Could you check a few things on this drawing? It's one solid part, dimensions in mm from its lowest x, y, z. A direction names the side the tool comes from. Round coordinates to 2 decimals unless told otherwise and drop trailing zeros. Loops run counter-clockwise (first coordinate to the right, second up) from the corner with the lowest first, then second, coordinate; pieces in that order, holes last. Notation, with made-up numbers: (49, 66) -> (75, 66) arc R24 ccw to (75, 81) -> close; hole circle Ø7 at (2.5, -30.75). An arc over 180 degrees is marked (long way). Write each question's results on one line, items separated by ' | '.
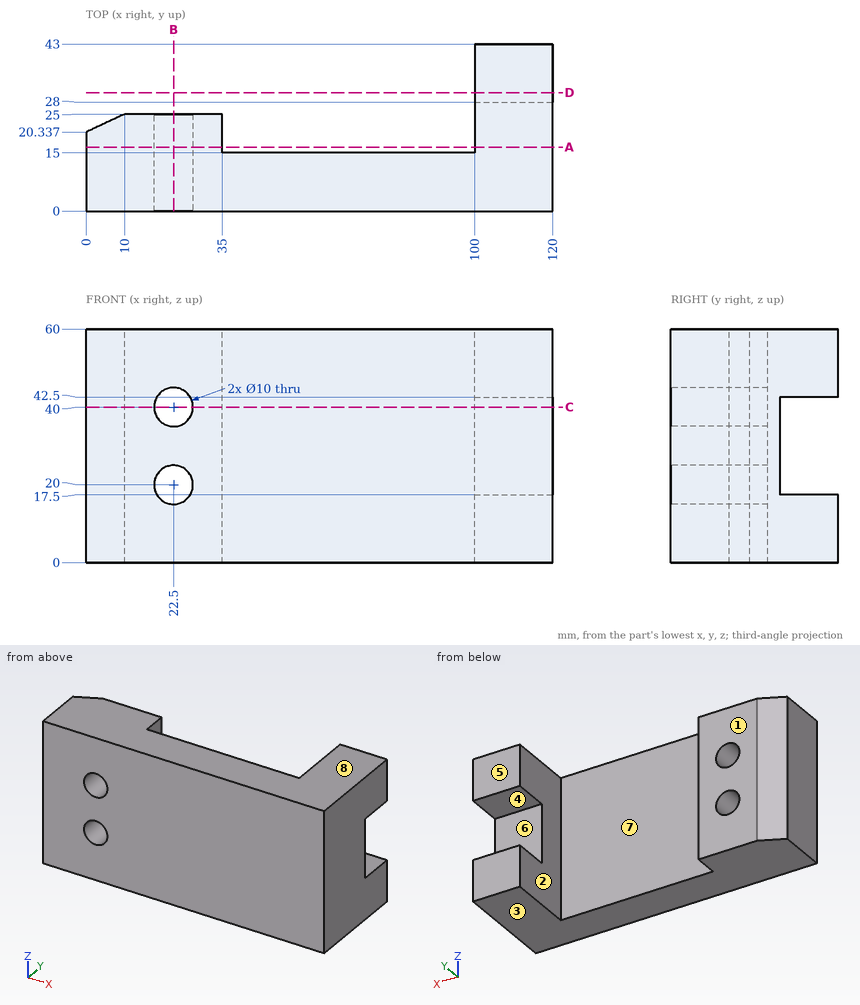
1) I want a section at C-C, the plane z = 40. Write out the boundary of the cut face in (x, y), plus the area to 3 significant figures.
Model answer:
outline: (0, 0) -> (17.5, 0) -> (17.5, 25) -> (10, 25) -> (0, 20.34) -> close; (27.5, 0) -> (120, 0) -> (120, 28) -> (100, 28) -> (100, 15) -> (35, 15) -> (35, 25) -> (27.5, 25) -> close | area: 2,140 mm2
2) I'm going to push flat-ended pins straight in: pin 1 (1.5 mm diameter, centred on x = 91.5, z = 8, fed in from +Y); pin 2 (5 mm diameter, centred on y = 6, z = 11.5, fed in from -X); pin 3 (14 mm diameter, centred on y = 27.5, z = 40, fed in from -X); pin 4 (10 mm diameter, centred on x = 111, z = 32.5, fed in from +Y). Where does each tip first touch, or does it pass through?
Model answer:
pin 1: stops at y = 15 | pin 2: stops at x = 0 | pin 3: stops at x = 0.35 | pin 4: stops at y = 28
3) If we mould it in two halves opening along Z, with no side actions, what happens to the marked faces 6, 7 and 8? For each: released by +Z, released by -Z, zero draft, split by the parting line, or undercut.
Model answer:
face 6: undercut | face 7: zero draft | face 8: released by +Z
4) I need wall thicknesses on line 1 (Z direction, x = 22, y = 9) (3 decimals); line 2 (X direction, y = 17.75, z = 20); line 3 (X direction, y = 14.25, z = 20). Which ranges of each line are inside material? Lowest first, please.
Model answer:
line 1: z = 0 to 15.025, 24.975 to 35.025, 44.975 to 60 | line 2: x = 0 to 17.5, 27.5 to 35, 100 to 120 | line 3: x = 0 to 17.5, 27.5 to 120
5) I want a section at D-D, the plane y = 30.5. Write out the boundary of the cut face in (x, z), plus the area to 3 significant figures.
Model answer:
outline: (100, 0) -> (120, 0) -> (120, 17.5) -> (100, 17.5) -> close; (100, 42.5) -> (120, 42.5) -> (120, 60) -> (100, 60) -> close | area: 700 mm2
6) I want a section at A-A, the plane y = 16.5. Write out the boundary of the cut face in (x, z), plus the area to 3 significant figures.
Model answer:
outline: (0, 0) -> (35, 0) -> (35, 60) -> (0, 60) -> close; (100, 0) -> (120, 0) -> (120, 60) -> (100, 60) -> close; hole circle Ø10 at (22.5, 20); hole circle Ø10 at (22.5, 40) | area: 3,140 mm2
7) I want a section at B-B, the plane x = 22.5. Write out the boundary of the cut face in (y, z), plus the area to 3 significant figures.
Model answer:
outline: (0, 0) -> (25, 0) -> (25, 15) -> (0, 15) -> close; (0, 25) -> (25, 25) -> (25, 35) -> (0, 35) -> close; (0, 45) -> (25, 45) -> (25, 60) -> (0, 60) -> close | area: 1,000 mm2
8) For the marked faces 1, 2, 3, 4 and 5, which set-ups out of +Z, -Z, +X, -X, +Y, -Y let a thin tool reach every point of the face, with its end or its side?
Model answer:
face 1: +Z, -Z, -X, +Y | face 2: +Z, -Z, +Y | face 3: -Z, +X, -X, +Y, -Y | face 4: +X, -X, +Y | face 5: +Z, -Z, +X, -X, +Y
